Geometry check sheet. Reference: the model listing, model coordinates, mm. A direction names the side the tool comes from. Coordinates: 2 decimals unless noted, no trailing zeros. Write each loop counter-clockwise with the first axis right and the second up, starting at its lowest first coordinate (ties: lowest second). Pieces come first, ordered by that corner, then holes. Notation, with made-up numbers: M -36.75,-27 L 5.25,-27 A33 cw 5.25,3 Z; hole C 78,4.25 d11. An arc over 180 degrees is marked long. Put each result on its own line as item: value. Start each with the question number.
1) Gauge pin test, flat ends, axial feed: pin 1 (5 mm diameter, centred on x = 103.5, z = -87, fed in from -Y); pin 2 (1 mm diameter, centred on y = -35.5, z = 24.5, fed in from +X); pin 3 (21 mm diameter, centred on y = -82.5, z = 70, fed in from +X). Record the tip position at first contact, or that the pin passes through.
2) Set-up check for faces 4 (the flat face through (-27, -63, -127.899)), 5 (the flat face through (123.256, -63, 53)), 6 (the flat face through (-3, -63, 43.378)), 7 (the flat face through (-89, -63, 81.651)), 8 (the flat face through (-126.963, -63, -118)): record each of +Z, -Z, +X, -X, +Y, -Y from which the full face is reachable in a straight line by a thin tool's end or side.
3) Cross-section at C-C on x = 38.5. Record the cut outline in (y, z), plus the area to 3 significant figures.
4) Cross-section at B-B on z = -123. Record the cut outline in (x, y).
5) Cross-section at A-A on y = -24.5. Record the cut outline in (x, z), plus the area to 3 significant figures.
6) Scan lines: line 1 along X through (y, z) = (-14.5, -61); line 2 along Y through (x, z) = (-78.5, -90); line 3 along Z through (x, y) = (95.5, -100). Record each from-to range of solid material in increasing order.
7) Mould release check, pull along X, two halves, no side actions. Record for faces 1 (the flat face through (86, -63, -147.122)), 2 (the flat face through (95.287, -63, -53)), 3 (the flat face through (76.237, -63, -32)): released by +X, released by -X, zero draft, split by the parting line, or undercut.
8) Cross-section at D-D on z = -87. Record the cut outline in (x, y), plus the area to 3 significant figures.
from build123d import *

# Parameters (mm, degrees)
F1_DEPTH = 127
F2_W     = 360.047168
F2_H     = 254
F3_DEPTH = 19.05


with BuildPart() as f1:
    # F0 (on Front) → F1 (new body)
    with BuildSketch(Plane.XZ):
        Polygon((-79.94371, 81.650516), (-98.99371, 81.650516), (-98.99371, -108.849484), (-79.94371, -108.849484), (-79.94371, 43.378164), (-79.94371, 62.428164), align=None)
        Polygon((123.25629, 62.428164), (-79.94371, 62.428164), (-79.94371, 43.378164), (76.237486, 43.378164), (95.287486, 43.378164), (123.25629, 43.378164), align=None)
        Polygon((76.237486, 43.378164), (76.237486, -108.849484), (76.237486, -127.899484), (76.237486, -147.121836), (95.287486, -147.121836), (95.287486, 43.378164), align=None)
        Polygon((-79.94371, -108.849484), (-98.99371, -108.849484), (-126.962514, -108.849484), (-126.962514, -127.899484), (76.237486, -127.899484), (76.237486, -108.849484), align=None)
    extrude(amount=F1_DEPTH)

    # F2 (on face) → F3 (join)
    with BuildSketch(Plane(origin=(0, 0, 0), x_dir=(-1, 0, 0), z_dir=(0, 1, 0))):
        with Locations((8.068025, -33.890009)):
            Rectangle(F2_W, F2_H)
    extrude(amount=F3_DEPTH)


solid = f1.part
Answer key:
1. pin 1: stops at y = 0
1. pin 2: stops at x = 95.29
1. pin 3: stops at x = 123.26
2. face 4: -Z, -X, -Y
2. face 5: +Z, -Z, +X, -Y
2. face 6: -Y
2. face 7: +Z, +X, -X, -Y
2. face 8: +Z, -Z, -X, -Y
3. outline: M -127,-127.9 L 0,-127.9 L 0,-160.89 L 19.05,-160.89 L 19.05,93.11 L 0,93.11 L 0,62.43 L -127,62.43 L -127,43.38 L 0,43.38 L 0,-108.85 L -127,-108.85 Z
3. area: 9,680 mm²
4. outline: M -188.09,0 L -126.96,0 L -126.96,-127 L 95.29,-127 L 95.29,0 L 171.96,0 L 171.96,19.05 L -188.09,19.05 Z
5. outline: M -126.96,-127.9 L 76.24,-127.9 L 76.24,-147.12 L 95.29,-147.12 L 95.29,43.38 L 123.26,43.38 L 123.26,62.43 L -79.94,62.43 L -79.94,81.65 L -98.99,81.65 L -98.99,-108.85 L -126.96,-108.85 Z; hole M -79.94,-108.85 L 76.24,-108.85 L 76.24,43.38 L -79.94,43.38 Z
5. area: 15,000 mm²
6. line 1: x = -98.99 to -79.94, 76.24 to 95.29
6. line 2: y = 0 to 19.05
6. line 3: z = 43.38 to 62.43
7. face 1: zero draft
7. face 2: released by +X
7. face 3: undercut
8. outline: M -188.09,0 L -98.99,0 L -98.99,-127 L -79.94,-127 L -79.94,0 L 76.24,0 L 76.24,-127 L 95.29,-127 L 95.29,0 L 171.96,0 L 171.96,19.05 L -188.09,19.05 Z
8. area: 11,700 mm²
